Autodesk Inventor part; units mm, degrees
ref_plane "YZ Plane" through (0, 0, 0) normal (1, 0, 0) x (0, 1, 0)
ref_plane "XZ Plane" through (0, 0, 0) normal (0, 1, 0) x (-1, 0, 0)
ref_plane "XY Plane" through (0, 0, 0) normal (0, 0, 1) x (1, 0, 0)
sketch "Sketch1" plane through (0, 0, 0) normal (0, 1, 0) x (-1, 0, 0)
  circle A0 centre (0, 0) radius 304.8
  dimension "d0" = 609.6
extrude "Extrusion1" add sketch "Sketch1" along normal blind 3.175
sketch "Sketch2" plane through (0, 3.175, 0) normal (0, 1, 0) x (1, 0, 0)
  circle A0 centre (0, 0) radius 304.8
  circle A1 centre (0, 0) radius 6.35
  dimension "d3" = 12.7
extrude "Extrusion2" cut sketch "Sketch2" against normal blind 3.175 contours A1
sketch "Sketch3" plane through (0, 3.175, 0) normal (0, 1, 0) x (1, 0, 0)
  circle A0 centre (0, 0) radius 6.35
  circle A1 centre (0, 292.1) radius 4.6302
  dimension "d6" = 292.1
hole "Hole1" at (0, 3.175, -292.1) direction (0, -1, 0) diameter 4.4958 end through all countersink diameter 8.4328 countersink angle 82
pattern_circular "Circular Pattern1" count 4 over 360 about axis through (0, 3.175, 0) along (0, -1, 0) of "Hole1"
sketch "Sketch11" plane through (0, 3.175, 0) normal (0, 1, 0) x (1, 0, 0)
  circle A0 centre (0, 0) radius 57.15 construction
  point P0 (0, 57.15)
  point P1 (57.15, 0)
  point P2 (0, -57.15)
  point P3 (-57.15, 0)
  dimension "d98" = 114.3
hole "Hole8" at (0, 3.175, -57.15) at (57.15, 3.175, 0) at (0, 3.175, 57.15) at (-57.15, 3.175, 0) direction (0, -1, 0) diameter 4.917 end through all
properties part number "2f1bd" material "Aluminum 6061"
Read the model definition and answer for the solid it produces. Units are mm, in the model's axes. Coordinates: 2 decimals unless noted, no trailing zeros. Write each loop counter-clockwise with the first axis right and the second up, starting at its lowest first coordinate (ties: lowest second). Pieces come first, ordered by that corner, then holes. Notation, with made-up numbers: (52.5, -14) -> (89.5, -14) arc R27 ccw to (89.5, 7) -> close; hole circle Ø1 at (-29.75, 69.5). An arc over 180 degrees is marked (long way). Return JSON: item names as keys, results as strings.
(1) Consider line 1 along Z through (x, y) = (0, 1.25); line 2 along Z through (x, y) = (57.15, 1.4); line 3 along X through (y, z) = (0.4, 100). Determine where each line is inside the solid, lowest interval first. Write a range as from..to.
Answers below:
{"line 1": "-304.8..-294.64, -289.56..-59.61, -54.69..-6.35, 6.35..54.69, 59.61..289.56, 294.64..304.8", "line 2": "-299.39..-2.46, 2.46..299.39", "line 3": "-287.93..287.93"}
(2) The part is cut by section B-B on z = 93. Give the vertices of the cut face in (x, y) (3 decimals), then the cut area to 3 significant figures.
Answers below:
{"outline": "(-290.265, 0) -> (290.265, 0) -> (290.265, 3.175) -> (-290.265, 3.175) -> close", "area": "1,840 mm^2"}
(3) The part is cut by section C-C on x = -200. Give the vertices of the cut face in (y, z) (3 decimals).
Answers below:
{"outline": "(0, -230.007) -> (3.175, -230.007) -> (3.175, 230.007) -> (0, 230.007) -> close"}
(4) The part is cut by section A-A on y = 2.3. State how many separate pieces and enclosed holes the cut face has, then the cut area to 3 significant figures.
Answers below:
{"separate pieces": "1", "enclosed holes": "9", "area": "292,000 mm^2"}
